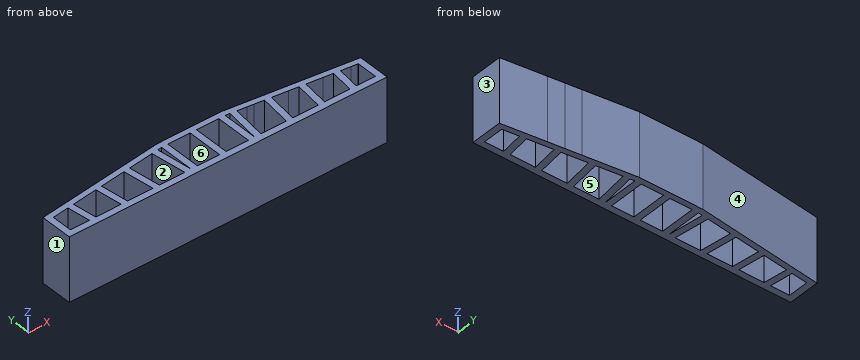
```python
from build123d import *

# Parameters (mm, degrees)
SKETCH1_W           = 7
SKETCH1_H           = 11.231344736
BOSS_EXTRUDE1_DEPTH = 20


with BuildPart() as part:
    # Sketch1 → Boss-Extrude1 (new body)
    with BuildSketch(Plane.XY):
        Polygon((-50, 0), (-8.117664451, 0), (50, 0), (50, 10), (36.215384615, 11.723076923), (31.292307692, 12.338461538), (26.369230769, 12.953846154), (10, 15), (-10, 15), (-50, 10), align=None)
        Polygon((-42.015564437, 2), (-48, 2), (-48, 8.481344736), (-42.905336644, 9.118177656), align=None, mode=Mode.SUBTRACT)
        Polygon((-40.920780891, 9.366247125), (-33.059182798, 10.348946887), (-32.015564437, 2), (-40, 2), align=None, mode=Mode.SUBTRACT)
        Polygon((-31.074627044, 10.597016356), (-23.213028952, 11.579716117), (-22.015564437, 2), (-30, 2), align=None, mode=Mode.SUBTRACT)
        Polygon((-21.228473198, 11.827785587), (-13.366875106, 12.810485348), (-12.015564437, 2), (-20, 2), align=None, mode=Mode.SUBTRACT)
        Polygon((15, 2), (12.015564437, 2), (13.366875106, 12.810485348), (16.305396275, 12.443170202), (18.289952029, 12.195100733), (21.228473198, 11.827785587), (20, 2), (17.015564437, 2), align=None, mode=Mode.SUBTRACT)
        Polygon((47.828413567, 8.502793041), (48, 8.481344736), (48, 2), (47.015564437, 2), (45, 2), (42.015564437, 2), (42.905336644, 9.118177656), (45.843857814, 8.75086251), align=None, mode=Mode.SUBTRACT)
        Polygon((37.015564437, 2), (32.015564437, 2), (33.059182798, 10.348946887), (37.982259721, 9.733562271), (40.920780891, 9.366247125), (40, 2), align=None, mode=Mode.SUBTRACT)
        Polygon((27.015564437, 2), (22.015564437, 2), (23.213028952, 11.579716117), (28.136105875, 10.964331502), (31.074627044, 10.597016356), (30, 2), align=None, mode=Mode.SUBTRACT)
        Polygon((-10, 2), (-11.382319352, 13.058554817), (-10, 13.231344736), align=None, mode=Mode.SUBTRACT)
        with Locations((-4.5, 7.615672368)):
            Rectangle(SKETCH1_W, SKETCH1_H, mode=Mode.SUBTRACT)
        with Locations((4.5, 7.615672368)):
            Rectangle(SKETCH1_W, SKETCH1_H, mode=Mode.SUBTRACT)
        Polygon((10, 2), (10, 13.231344736), (11.382319352, 13.058554817), align=None, mode=Mode.SUBTRACT)
    extrude(amount=BOSS_EXTRUDE1_DEPTH)


solid = part.part
```
Source: CAD feature listing. Evaluate the final solid. Frame: model axes, mm. Face numbers are marked on the shaded views. A direction names the side the tool comes from. Give positions to 0.01 mm unless a question says otherwise; leave off trailing zeros. Loops run counter-clockwise (first coordinate to the right, second up) from the corner with the lowest first, then second, coordinate; pieces in that order, holes last. Notation, with made-up numbers: M 32.25,5.5 L 48.25,5.5 A28 cw 48.25,37.5 Z; hole C -22.75,-38.75 d1. An arc over 180 degrees is marked long. Put each result on its own line as item: value.
Q1. Mould query, pull axis X, two halves, no side actions, for the marked faces 3, 4, 5 and 6. Classes: released by +X, released by -X, zero draft, split by the parting line, or undercut.
Response values:
face 3: released by +X
face 4: released by -X
face 5: undercut
face 6: undercut
Q2. Pin query (flat end, axial travel): P1, Ø5, axis at x = 44.5, z = 15, coming from the +Y side; P2, Ø4, axis at x = 25.5, z = 6.5, coming from the +Y side; P3, Ø4, axis at x = -34.5, z = 9, coming from the +Y side. Return the tip coordinate at first contact, or that it passes through.
Response values:
P1: stops at y = 11
P2: stops at y = 13.31
P3: stops at y = 12.19
Q3. Section B-B (z = 13.5). Count the separate pieces of the cut face and the enclosed holes in it, and give its area (3 significant figures).
Response values:
separate pieces: 1
enclosed holes: 12
area: 616 mm²
Q4. Line query: probe 1 along Y at (x, z) = (-44.5, 9); probe 2 along Y at (x, z) = (46, 5). Output: solid intervals per line, ascending. Write a range as [from, to].
Response values:
probe 1: y = [0, 2], [8.92, 10.69]
probe 2: y = [0, 2], [8.73, 10.5]
Q5. Section A-A (x = 15). Return the cut outline in (y, z) (3 decimals), and give its area (3 significant figures).
Response values:
outline: M 0,0 L 2,0 L 2,20 L 0,20 Z; M 12.606,0 L 14.375,0 L 14.375,20 L 12.606,20 Z
area: 75.4 mm²
Q6. Reachability of the marked faces 1 and 2 from +Z, -Z, +X, -X, +Y, -Y: full face, straight path, thin tool, end or side. Return the list, or none.
Response values:
face 1: +Z, -Z, -X, +Y, -Y
face 2: +Z, -Z
